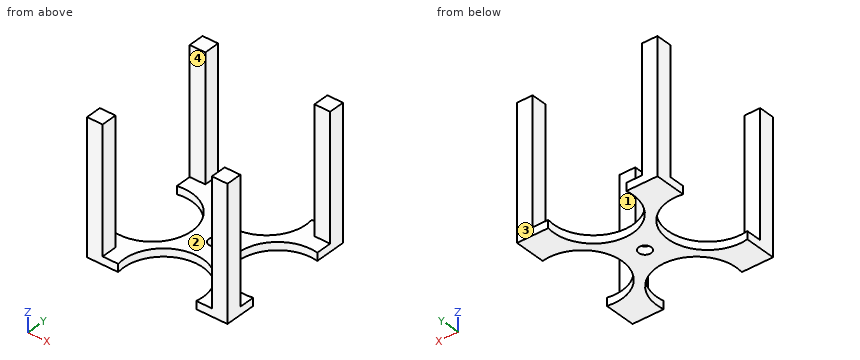
from build123d import *

# Parameters (mm, degrees)
F0_W     = 114.3
F0_H     = 114.3
F1_DEPTH = 6.35
F3_R     = 5.08
F4_DEPTH = 25.4
F2_W     = 12.7
F2_H     = 12.7
F5_DEPTH = 101.6
F7_DEPTH = 107.951


with BuildPart() as f1:
    # F0 (on Top) → F1 (new body)
    with BuildSketch(Plane.XY):
        Rectangle(F0_W, F0_H)
    extrude(amount=F1_DEPTH)

    # F3 (on face) → F4 (cut)
    with BuildSketch(Plane.XY.offset(6.35)):
        Circle(F3_R)
    extrude(amount=-F4_DEPTH, mode=Mode.SUBTRACT)

    # F2 (on face) → F5 (join)
    with BuildSketch(Plane.XY.offset(6.35)):
        with Locations((50.8, 50.8)):
            Rectangle(F2_W, F2_H)
        with Locations((-50.8, 50.8)):
            Rectangle(F2_W, F2_H)
        with Locations((-50.8, -50.8)):
            Rectangle(F2_W, F2_H)
        with Locations((50.8, -50.8)):
            Rectangle(F2_W, F2_H)
    extrude(amount=F5_DEPTH)

    # F6 (on face) → F7 (cut, through all)
    with BuildSketch(Plane(origin=(0, 0, 0), x_dir=(1, 0, 0), z_dir=(0, 0, -1))):
        with BuildLine():
            Line((-57.15, 31.75), (-57.15, -31.75))
            ThreePointArc((-57.15, -31.75), (-18.698453, 0), (-57.15, 31.75))
        make_face()
        with BuildLine():
            Line((-31.75, -57.15), (31.75, -57.15))
            ThreePointArc((31.75, -57.15), (0, -18.698453), (-31.75, -57.15))
        make_face()
        with BuildLine():
            Line((57.15, -31.75), (57.15, 31.75))
            ThreePointArc((57.15, 31.75), (18.698453, 0), (57.15, -31.75))
        make_face()
        with BuildLine():
            Line((31.75, 57.15), (-31.75, 57.15))
            ThreePointArc((-31.75, 57.15), (0, 18.698453), (31.75, 57.15))
        make_face()
    extrude(amount=-F7_DEPTH, mode=Mode.SUBTRACT)


solid = f1.part
Build history of the part. All positions in model axes, mm. Face numbers are marked on the shaded views. A direction names the side the tool comes from. Coordinates: 2 decimals unless noted, no trailing zeros. Order: outer loops, then holes, each group sorted by start corner. A loop starts at its lowest first (then second) coordinate and runs counter-clockwise, first axis right, second up. Notation, with made-up numbers: (-1, 72.25) - (34, 72.25) arc R19 cw to (34, 77.25) - close; hole circle Ø4 at (55.25, 67.25). An arc over 180 degrees is marked (long way). Put each result on its own line as item: value.
1. Tool access for the marked faces 3 and 4: list every direction of +Z, -Z, +X, -X, +Y, -Y with a clear straight run to the whole face (end or side of a thin tool).
Answer sheet:
face 3: +Z, -Z, +X, -X, +Y
face 4: +Z, +X, -X
2. Saw through at B-B (x = 0). Write the cut outline in (y, z).
Answer sheet:
outline: (-18.7, 0) - (-5.08, 0) - (-5.08, 6.35) - (-18.7, 6.35) - close; (5.08, 0) - (18.7, 0) - (18.7, 6.35) - (5.08, 6.35) - close
3. Drop a flat-ended pin along its axis: P1, Ø1.5, axis at x = -36, y = 29, coming from the -Z side. Give the stop position or say it passes through.
Answer sheet:
P1: stops at z = 0
4. Pull direction X, two halves, no side cores. Call the marked faces 1 and 2: pulls with the +X half, pulls with the -X half, needs draft (parallel to the pull), parting line crosses it, or undercut.
Answer sheet:
face 1: needs draft
face 2: undercut
5. Saw through at A-A (z = 36.5). Write the cut outline in (x, y), and give its area (3 significant figures).
Answer sheet:
outline: (-57.15, -57.15) - (-44.45, -57.15) - (-44.45, -44.45) - (-57.15, -44.45) - close; (-57.15, 44.45) - (-44.45, 44.45) - (-44.45, 57.15) - (-57.15, 57.15) - close; (44.45, -57.15) - (57.15, -57.15) - (57.15, -44.45) - (44.45, -44.45) - close; (44.45, 44.45) - (57.15, 44.45) - (57.15, 57.15) - (44.45, 57.15) - close
area: 645 mm^2
6. Probe line 1 along X through (y, z) = (-48, 38.5); line 2 along Z through (x, y) = (-6, -19). List the from-to ranges inside material, lowest first. Write a range as [from, to].
Answer sheet:
line 1: x = [-57.15, -44.45], [44.45, 57.15]
line 2: z = [0, 6.35]
7. Saw through at D-D (y = 13). Write the cut outline in (x, z).
Answer sheet:
outline: (-21.43, 0) - (21.43, 0) - (21.43, 6.35) - (-21.43, 6.35) - close
